Design review of the part shown in the three views and the two pictorial views. Dimensions are in mm from the part's minimum x, y and z. A direction names the side the tool comes from. Give positions to 0.01 mm unless a question says otherwise; leave off trailing zeros. Loops run counter-clockwise (first coordinate to the right, second up) from the corner with the lowest first, then second, coordinate; pieces in that order, holes last. Notation, with made-up numbers: (37.5, 65) - (66.5, 65) arc R21 ccw to (66.5, 79) - close; hole circle Ø11 at (-39, 87). An arc over 180 degrees is marked (long way). Answer in a Markdown table with one row per item.
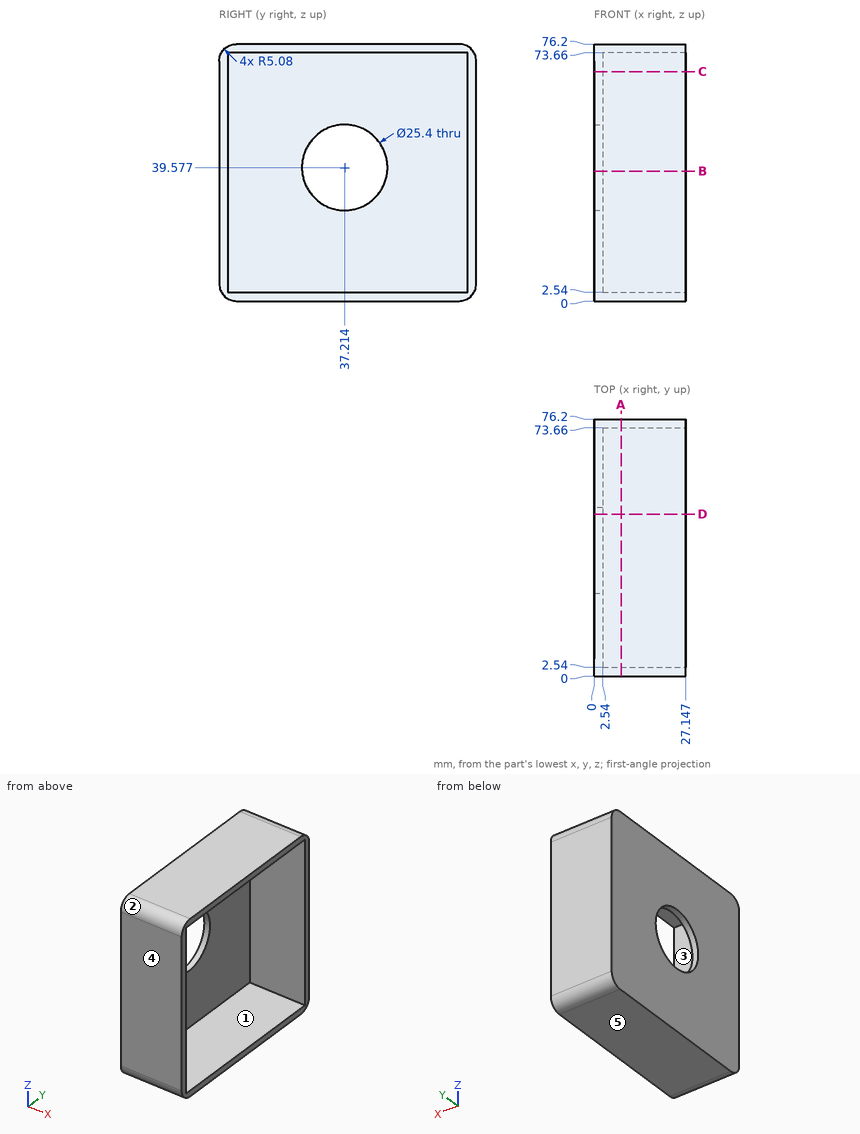
1. Mouldability with a two-part tool opening along Z and no side actions: class the marked faces 3, 4 and 5 as released by +Z, released by -Z, zero draft, split by the parting line, or undercut.
Values:
| item | result |
|---|---|
| face 3 | undercut |
| face 4 | zero draft |
| face 5 | released by -Z |
2. We need section D-D, the plane y = 48. Give the boundary of the cut face in (x, z).
Values:
| item | result |
|---|---|
| outline | (0, 0) - (27.15, 0) - (27.15, 2.54) - (2.54, 2.54) - (2.54, 32.87) - (0, 32.87) - close; (0, 46.28) - (2.54, 46.28) - (2.54, 73.66) - (27.15, 73.66) - (27.15, 76.2) - (0, 76.2) - close |
3. We need section A-A, the plane x = 8. Give the boundary of the cut face in (y, z).
Values:
| item | result |
|---|---|
| outline | (0, 5.08) arc R5.08 ccw to (5.08, 0) - (71.12, 0) arc R5.08 ccw to (76.2, 5.08) - (76.2, 71.12) arc R5.08 ccw to (71.12, 76.2) - (5.08, 76.2) arc R5.08 ccw to (0, 71.12) - close; hole (2.54, 2.54) - (73.66, 2.54) - (73.66, 73.66) - (2.54, 73.66) - close |
4. For the marked faces 1 and 2, list the 3-axis set-ups (+Z, -Z, +X, -X, +Y, -Y) from which the entire face can be reached by the end or side of a thin tool; tool diameter is ignored.
Values:
| item | result |
|---|---|
| face 1 | +X |
| face 2 | +Z, +X, -X, -Y |
5. We need section B-B, the plane z = 38.5. Give the boundary of the cut face in (x, y).
Values:
| item | result |
|---|---|
| outline | (0, 0) - (27.15, 0) - (27.15, 2.54) - (2.54, 2.54) - (2.54, 24.56) - (0, 24.56) - close; (0, 49.87) - (2.54, 49.87) - (2.54, 73.66) - (27.15, 73.66) - (27.15, 76.2) - (0, 76.2) - close |
6. Clearance check with flat-ended pins moving along their axes: pin 1 (2 mm diameter, centred on x = 15.5, z = 19, fed in from -Y); pin 2 (15 mm diameter, centred on y = 37.21, z = 39.58, fed in from +X); pin 3 (21.5 mm diameter, centred on y = 43, z = 46, fed in from +X). State where each tip first meets the part, or that it passes through.
Values:
| item | result |
|---|---|
| pin 1 | stops at y = 0 |
| pin 2 | passes through |
| pin 3 | stops at x = 2.54 |
7. We need section C-C, the plane z = 68. Give the boundary of the cut face in (x, y).
Values:
| item | result |
|---|---|
| outline | (0, 0) - (27.15, 0) - (27.15, 2.54) - (2.54, 2.54) - (2.54, 73.66) - (27.15, 73.66) - (27.15, 76.2) - (0, 76.2) - close |
8. Wall thickness on line 1 (Z direction, x = 12.25, y = 50); line 2 (X direction, y = 34, z = 61.5): over which ranges is each line inside the solid? List them lowest first. Write a range as [from, to].
Values:
| item | result |
|---|---|
| line 1 | z = [0, 2.54], [73.66, 76.2] |
| line 2 | x = [0, 2.54] |
